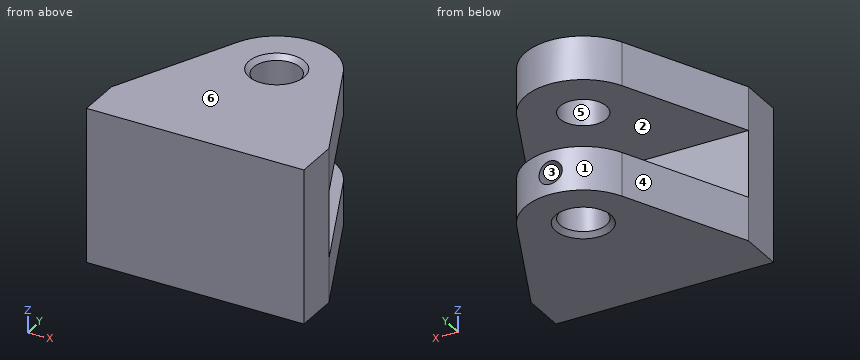
from build123d import *

# Parameters (mm, degrees)
P_IDAT_VYSUNUT_M1_DEPTH       = 15
SKICA4_W                      = 75
SKICA4_H                      = 14.99699372
P_IDAT_VYSUNUT_M2_DEPTH       = 11.5
SKICA6_R                      = 8
ODEBRAT_VYSUNUT_M1_DEPTH      = 54
ODEBRAT_VYSUNUT_M2_REACH      = 71
ODEBRAT_VYSUNUT_M2_END_RADIUS = 8
SKICA7_R                      = 4
ZKOSEN_1_SIZE                 = 1.6


with BuildPart() as part:
    # Skica1 → Přidat vysunutím1 (new body)
    with BuildSketch(Plane.XY):
        with BuildLine():
            Line((-37.5, 0), (-37.5, 14.99699372))
            Line((-37.5, 14.99699372), (-18.194945848, 57.300242817))
            ThreePointArc((-18.194945848, 57.300242817), (0, 68.99699372), (18.194945848, 57.300242817))
            Line((18.194945848, 57.300242817), (37.5, 14.99699372))
            Line((37.5, 14.99699372), (37.5, 0))
            Line((37.5, 0), (-37.5, 0))
        make_face()
    extrude(amount=P_IDAT_VYSUNUT_M1_DEPTH)

    # Skica4 → Přidat vysunutím2 (add)
    with BuildSketch(Plane(origin=(0, 0, 0), x_dir=(-1, 0, 0), z_dir=(0, 0, -1))):
        with Locations((0, 7.49849686)):
            Rectangle(SKICA4_W, SKICA4_H)
    extrude(amount=P_IDAT_VYSUNUT_M2_DEPTH)

    # Zrcadlit1: part across plane


with BuildPart() as part_1:
    add(part.part)
    add(part.part.mirror(Plane.XY.offset(-11.5)))

    # Skica6 → Odebrat vysunutím1 (cut, through all)
    with BuildSketch(Plane.XY.offset(15)):
        with Locations((0, 49)):
            Circle(SKICA6_R)
    extrude(amount=-ODEBRAT_VYSUNUT_M1_DEPTH, mode=Mode.SUBTRACT)

    # Odebrat vysunutím2: up to this cylinder (the profile starts outside it)
    odebrat_vysunut_m2_end = Plane(origin=(0, 49, -30.5), z_dir=(0, 0, 1)) * Cylinder(ODEBRAT_VYSUNUT_M2_END_RADIUS, 159, mode=Mode.PRIVATE)
    # Skica7 → Odebrat vysunutím2 (cut, up to the surface)
    with BuildSketch(Plane(origin=(0, 69, 0), x_dir=(1, 0, 0), z_dir=(0, 1, 0)), mode=Mode.PRIVATE) as odebrat_vysunut_m2_sk1:
        with Locations(Location((0, 30.5, 0), (0, 0, 270))):  # turned: the seam where the file's is
            Circle(SKICA7_R)
    odebrat_vysunut_m2_tool1 = extrude(odebrat_vysunut_m2_sk1.sketch, amount=-ODEBRAT_VYSUNUT_M2_REACH, mode=Mode.PRIVATE) - odebrat_vysunut_m2_end
    add(odebrat_vysunut_m2_tool1.solids().sort_by_distance((0, 69, -30.5))[0], mode=Mode.SUBTRACT)

    # Zkosení1
    zkosen_1_edges = [part_1.edges().sort_by_distance(p)[0] for p in [
        (-8, 49, -38),
        (-8, 49, 15),
    ]]
    chamfer(zkosen_1_edges, length=ZKOSEN_1_SIZE)


solid = part_1.part
Check sheet for the modelled part. Datum: model origin and axes. Units: mm. Face numbers are marked on the shaded views. A direction names the side the tool comes from. Round coordinates to 2 decimals unless told otherwise and drop trailing zeros. Order: outer loops, then holes, each group sorted by start corner. A loop starts at its lowest first (then second) coordinate and runs counter-clockwise, first axis right, second up.
(1) Cross-section at B-B, the plane z = 2. Enter the section's corners in (x, y).
(2) Draft check along X on the marked faces 4, 5 and 6. Enter one of: pulls with the +X half, pulls with the -X half, needs draft (parallel to the pull), parting line crosses it, or undercut.
(3) Cross-section at C-C, the plane y = 64.5. Enter the section's corners in (x, z), and give its area (3 significant figures).
(4) Scan lines: probe 1 along Z at (x, y) = (0, 62); probe 2 along Z at (x, y) = (6.5, 32); probe 3 along X at (y, z) = (61.75, -30.5). Record each from-to range of solid material in increasing order.
(5) Cross-section at A-A, the plane x = 0. Enter the section's corners in (y, z).
(6) Access from +Z, -Z, +X, -X, +Y, -Y to the whole of each face (thin tool, end or side, straight path). Record for the marked faces 1, 2 and 3.
(7) Go/stop test with flat-tipped pins: P1, Ø18.5, axis at x = 17.5, z = -6.5, coming from the +Y side; P2, Ø10, axis at y = 37, z = -3.5, coming from the +X side; P3, Ø5, axis at x = 0, z = -30.5, coming from the +Y side. Record where each tip stops, or that it passes through.
(8) Cross-section at D-D, the plane y = 19. Enter the section's corners in (x, z), and give its area (3 significant figures).
Check sheet entries:
1. outline: (-37.5, 0) - (37.5, 0) - (37.5, 15) - (18.19, 57.3) arc R20 ccw to (-18.19, 57.3) - (-37.5, 15) - close; hole circle Ø16 at (0, 49)
2. face 4: pulls with the -X half
2. face 5: undercut
2. face 6: needs draft
3. outline: (-12.64, -38) - (12.64, -38) - (12.64, -23) - (-12.64, -23) - close; (-12.64, 0) - (12.64, 0) - (12.64, 15) - (-12.64, 15) - close; hole circle Ø8 at (0, -30.5)
3. area: 708 mm2
4. probe 1: z = -38 to -34.5, -26.5 to -23, 0 to 15
4. probe 2: z = -38 to -23, 0 to 15
4. probe 3: x = -15.41 to -4, 4 to 15.41
5. outline: (0, -38) - (39.4, -38) - (41, -36.4) - (41, -23) - (15, -23) - (15, 0) - (41, 0) - (41, 13.4) - (39.4, 15) - (0, 15) - close; (57, -36.4) - (58.6, -38) - (69, -38) - (69, -34.5) - (57, -34.5) - close; (57, -26.5) - (69, -26.5) - (69, -23) - (57, -23) - close; (57, 0) - (69, 0) - (69, 15) - (58.6, 15) - (57, 13.4) - close
6. face 1: +Z, -Z, +Y
6. face 2: +X, -X, +Y
6. face 3: +Y
7. P1: stops at y = 65.75
7. P2: stops at x = 29.09
7. P3: stops at y = 41.4
8. outline: (-35.67, -38) - (35.67, -38) - (35.67, -23) - (-35.67, -23) - close; (-35.67, 0) - (35.67, 0) - (35.67, 15) - (-35.67, 15) - close
8. area: 2,140 mm2
